from build123d import *

# Parameters (mm, degrees)
F1_DEPTH = 31.75
F2_R     = 3.3782
F2_R_2   = 2.54
F3_DEPTH = 3.175


# Not quite as in the source:
# - a feature names something its author has since deleted; it is built from what else it names


with BuildPart() as f1:
    # F0 (on Front) → F1 (new body)
    with BuildSketch(Plane.XZ):
        Polygon((3.556, 2.0828), (-3.556, 2.0828), (-3.556, 0), (-7.4295, 0), (-7.4295, -2.032), (-2.54, -2.032), (-2.54, -5.334), (2.54, -5.334), (2.54, -2.032), (7.4295, -2.032), (7.4295, 0), (3.556, 0), align=None)
    extrude(amount=F1_DEPTH)

    # F2 (on face) → F3 (cut)
    with BuildSketch(Plane.XY.offset(2.0828)):
        with Locations((0, -21.3868)):
            Circle(F2_R)
        with Locations((0, -7.6454)):
            Circle(F2_R_2)
    extrude(amount=-F3_DEPTH, mode=Mode.SUBTRACT)


solid = f1.part
Verification items for the finished model (mm, model axes). A direction names the side the tool comes from. Round coordinates to 2 decimals unless told otherwise and drop trailing zeros. Loops run counter-clockwise (first coordinate to the right, second up) from the corner with the lowest first, then second, coordinate; pieces in that order, holes last. Notation, with made-up numbers: (44, 86.25) - (76, 86.25) arc R29 cw to (76, 119.25) - close; hole circle Ø1 at (81.25, 28.5). An arc over 180 degrees is marked (long way). Answer in a Markdown table with one row per item. Add a question column.
Q1. Release check for a two-part mould opening along X. For faces 1 (the face through (-3.556, -16, 1)), 2 (the face through (-0.44, -18.037, 0.518)), 3 (the face through (-5, -16, 0)) record: pulls with the +X half, pulls with the -X half, needs draft (parallel to the pull), parting line crosses it, or undercut.
Q2. Section check A-A on x = 0. Enter the section's corners in (y, z) (3 decimals), plus the area to 3 significant figures.
Q3. Section check B-B on y = -1.5. Enter the section's corners in (x, z), plus the area to 3 significant figures.
Q4. Section check C-C on z = -2.75. Enter the section's corners in (x, y), plus the area to 3 significant figures.
Q5. Section check D-D on z = -0.75. Enter the section's corners in (x, y).
Q6. Material ranges on line 1 (Y direction, x = 0, z = -0.3) (3 decimals); line 2 (Z direction, x = -6.75, y = -27); line 3 (Y direction, x = 2.75, z = 0), recorded low to high.
Q7. Gauge pin test, flat ends, axial feed: pin 1 (1 mm diameter, centred on y = -15.5, z = 1, fed in from +X); pin 2 (0.6 mm diameter, centred on y = -8.5, z = 1, fed in from -X); pin 3 (1.5 mm diameter, centred on x = -6, y = -9, fed in from -Z). Record the tip position at first contact, or that the pin passes through.
Q8. Tool access check on faces 4 (the face through (0, -8, -1.092)), 5 (the face through (6, -16, 0)), 6 (the face through (2.54, -16, -4)). Record the directions out of +Z, -Z, +X, -X, +Y, -Y that give a thin tool (end or side, any length) a straight path to the whole face; none if there is none.
Found:
| question | item | result |
|---|---|---|
| 1 | face 1 | pulls with the -X half |
| 1 | face 2 | undercut |
| 1 | face 3 | needs draft |
| 2 | outline | (-31.75, -5.334) - (0, -5.334) - (0, 2.083) - (-5.105, 2.083) - (-5.105, -1.092) - (-10.185, -1.092) - (-10.185, 2.083) - (-18.009, 2.083) - (-18.009, -1.092) - (-24.765, -1.092) - (-24.765, 2.083) - (-31.75, 2.083) - close |
| 2 | area | 198 mm² |
| 3 | outline | (-7.43, -2.03) - (-2.54, -2.03) - (-2.54, -5.33) - (2.54, -5.33) - (2.54, -2.03) - (7.43, -2.03) - (7.43, 0) - (3.56, 0) - (3.56, 2.08) - (-3.56, 2.08) - (-3.56, 0) - (-7.43, 0) - close |
| 3 | area | 61.8 mm² |
| 4 | outline | (-2.54, -31.75) - (2.54, -31.75) - (2.54, 0) - (-2.54, 0) - close |
| 4 | area | 161 mm² |
| 5 | outline | (-7.43, -31.75) - (7.43, -31.75) - (7.43, 0) - (-7.43, 0) - close; hole circle Ø6.76 at (0, -21.39); hole circle Ø5.08 at (0, -7.65) |
| 6 | line 1 | y = -31.75 to -24.765, -18.009 to -10.185, -5.105 to 0 |
| 6 | line 2 | z = -2.03 to 0 |
| 6 | line 3 | y = -31.75 to -23.35, -19.42 to 0 |
| 7 | pin 1 | stops at x = 3.56 |
| 7 | pin 2 | stops at x = -3.56 |
| 7 | pin 3 | stops at z = -2.03 |
| 8 | face 4 | +Z |
| 8 | face 5 | +Z, +X, +Y, -Y |
| 8 | face 6 | -Z, +X, +Y, -Y |
